from build123d import *
from build123d.topology import SkipClean

# Parameters (mm, degrees)
SKETCH3_W                 = 27
SKETCH3_H                 = 47.5
SKETCH3_R                 = 1.5
BOSS_EXTRUDE1_DEPTH       = 9
FILLET1_R                 = 2.5
SKETCH4_W                 = 26
SKETCH4_H                 = 44
BOSS_EXTRUDE5_DEPTH       = 15
SKETCH5_W                 = 25
SKETCH5_H                 = 18
BOSS_EXTRUDE6_DEPTH       = 5
SKETCH5_3_W               = 42
SKETCH5_3_H               = 18
SKETCH5_3_R               = 1
BOSS_EXTRUDE7_DEPTH       = 6
FILLET4_R                 = 2.5
CUT_EXTRUDE1_DEPTH        = 47.487229429
SKETCH6_5_R               = 22.5
BOSS_EXTRUDE8_DEPTH       = 26
SKETCH9_W                 = 7
SKETCH9_H                 = 15
SKETCH9_W_2               = 5
SKETCH9_H_2               = 6
BOSS_EXTRUDE9_DEPTH       = 7
SKETCH10_R                = 1
CUT_EXTRUDE2_DEPTH        = 41.437511922
BOSS_EXTRUDE10_DEPTH      = 5
BOSS_EXTRUDE10_DEPTH_BACK = 31
SKETCH6_6_R               = 5


with BuildPart() as part:
    # Sketch3 → Boss-Extrude1 (new body)
    with BuildSketch(Plane(origin=(0, 0, 0), x_dir=(1, 0, 0), z_dir=(0, 1, 0))):
        Rectangle(SKETCH3_W, SKETCH3_H)
        with Locations(Location((-11, 21.25, 0), (0, 0, 270))):
            Circle(SKETCH3_R, mode=Mode.SUBTRACT)
        with Locations(Location((11, 21.25, 0), (0, 0, 90))):
            Circle(SKETCH3_R, mode=Mode.SUBTRACT)
    extrude(amount=BOSS_EXTRUDE1_DEPTH)

    # Fillet1
    fillet1_edges = [part.edges().sort_by_distance(p)[0] for p in [
        (-13.5, 4.5, -23.75),
        (13.5, 4.5, -23.75),
    ]]
    fillet(fillet1_edges, radius=FILLET1_R)

    # Sketch4 → Boss-Extrude5 (add)
    with BuildSketch(Plane.XZ):
        Rectangle(SKETCH4_W, SKETCH4_H)
    extrude(amount=BOSS_EXTRUDE5_DEPTH)

    # Sketch5 → Boss-Extrude6 (add)
    with BuildSketch(Plane.XZ.offset(15)):
        with Locations((0, -0.75)):
            Rectangle(SKETCH5_W, SKETCH5_H)
    extrude(amount=-BOSS_EXTRUDE6_DEPTH)

    # Sketch5<3> → Boss-Extrude7 (add)
    with BuildSketch(Plane.XZ.offset(15)):
        with Locations((0, -0.75)):
            Rectangle(SKETCH5_3_W, SKETCH5_3_H)
        with Locations(Location((-18, -6.25, 0), (0, 0, 270))):
            Circle(SKETCH5_3_R, mode=Mode.SUBTRACT)
        with Locations(Location((18, -6.25, 0), (0, 0, 270))):
            Circle(SKETCH5_3_R, mode=Mode.SUBTRACT)
        with Locations(Location((-18, 4.75, 0), (0, 0, 270))):
            Circle(SKETCH5_3_R, mode=Mode.SUBTRACT)
        with Locations(Location((18, 4.75, 0), (0, 0, 270))):
            Circle(SKETCH5_3_R, mode=Mode.SUBTRACT)
    extrude(amount=BOSS_EXTRUDE7_DEPTH)

    # Fillet4
    fillet4_edges = [part.edges().sort_by_distance(p)[0] for p in [
        (21, -18, 8.25),
        (-21, -18, 8.25),
        (-21, -18, -9.75),
        (21, -18, -9.75),
    ]]
    fillet(fillet4_edges, radius=FILLET4_R)

    # Sketch6 → Cut-Extrude1 (cut, through all)
    with BuildSketch(Plane.ZY.offset(13)):
        with BuildLine():
            ThreePointArc((-16.66827394, -15), (-20.300466386, -7.910658998), (-21.234838924, 0))
            Line((-21.234838924, 0), (-22, 0))
            Line((-22, 0), (-22, -15))
            Line((-22, -15), (-16.66827394, -15))
        make_face()
        with BuildLine():
            Line((22, -15), (22, -9.995713029))
            ThreePointArc((22, -9.995713029), (20.719530361, -12.590758918), (19.116588355, -15))
            Line((19.116588355, -15), (22, -15))
        make_face()
    extrude(amount=-CUT_EXTRUDE1_DEPTH, mode=Mode.SUBTRACT)

    # Sketch6<5> → Boss-Extrude8 (add)
    with BuildSketch(Plane.ZY.offset(13)):
        with Locations((1.224157208, -1.357752838)):
            Circle(SKETCH6_5_R)
    extrude(amount=-BOSS_EXTRUDE8_DEPTH)

    # Sketch9 → Boss-Extrude9 (add)
    with BuildSketch(Plane.ZY.offset(13)):
        with Locations((2.25, 14)):
            Rectangle(SKETCH9_W, SKETCH9_H)
        with Locations((10.25, 9.5)):
            Rectangle(SKETCH9_W_2, SKETCH9_H_2)
    boss_extrude9 = extrude(amount=BOSS_EXTRUDE9_DEPTH)

    # Sketch10 → Cut-Extrude2 (cut, through all)
    with BuildSketch(Plane(origin=(0, 0, -1.25), x_dir=(-1, 0, 0), z_dir=(0, 0, -1))):
        with Locations((16.5, 9)):
            Circle(SKETCH10_R)
        with Locations((16.5, 19)):
            Circle(SKETCH10_R)
    cut_extrude2 = extrude(amount=-CUT_EXTRUDE2_DEPTH, mode=Mode.SUBTRACT)

    # Mirror1: Boss-Extrude9, Cut-Extrude2 across plane
    add(boss_extrude9.mirror(Plane(origin=(0, 0, 0), x_dir=(0, 0, 1), z_dir=(1, 0, 0))))
    add(cut_extrude2.mirror(Plane(origin=(0, 0, 0), x_dir=(0, 0, 1), z_dir=(1, 0, 0))), mode=Mode.SUBTRACT)

    # Sketch6<6> → Boss-Extrude10 (add, two sides: drawn at the far end of the back side and taken through both)
    with SkipClean():  # the faces are left unmerged after this step: merging them gives an invalid solid
        with BuildSketch(Plane.ZY.offset(13).offset(-BOSS_EXTRUDE10_DEPTH_BACK)):
            with Locations((1.224157208, -1.357752838)):
                Circle(SKETCH6_6_R)
        extrude(amount=BOSS_EXTRUDE10_DEPTH + BOSS_EXTRUDE10_DEPTH_BACK)


solid = part.part
Part model, mm, in its own coordinate system. A direction names the side the tool comes from. Coordinates: 2 decimals unless noted, no trailing zeros. Loops run counter-clockwise (first coordinate to the right, second up) from the corner with the lowest first, then second, coordinate; pieces in that order, holes last. Notation, with made-up numbers: (40.5, 0) -> (48.5, 0) arc R26 cw to (48.5, 29) -> close; hole circle Ø5 at (-21, -7). An arc over 180 degrees is marked (long way). Use a Markdown table: item, result. Add a question column.
Item 1: Probe probe 1 along Y at (x, z) = (16.5, 1.25); probe 2 along X at (y, z) = (-19.55, 4.75); probe 3 along Y at (x, z) = (-16.5, 2.75). List the from-to ranges inside material, lowest first.
Item 2: Band-saw the part on C-C on z = -12.5. Write the cut outline in (x, y).
Item 3: Which spindle directions (+Z, -Z, +X, -X, +Y, -Y) get a long thin tool onto all of the face, cutting with end or side? Do faces 5 (the flat face through (-16, 12.5, 10)), 6 (the cylindrical face through (-15.47, -6.24, 0.14)), 7 (the flat face through (-20, 14, 2)), 8 (the flat face through (16, -18, 8.25)). Say none if no direction does.
Item 4: Band-saw the part on D-D on y = -2. Write the cut outline in (x, z), plus the area to 3 significant figures.
Item 5: Pull direction Y, two halves, no side cores. Call faces 1 (the flat face through (16, 12.5, 10)), 2 (the flat face through (-20, 10, 10)), 3 (the flat face through (-13, -9, 1)), 4 (the flat face through (-17, -15, -1)): +Y half, -Y half, draft (parallel to the pull), parting line (faces both ways), or undercut.
Item 6: Flat gauge pins, fed straight in: P1, Ø12, axis at y = -1, z = -4.5, coming from the -X side; P2, Ø12, axis at y = 10.5, z = 2.5, coming from the +X side; P3, Ø5, axis at y = -2, z = 2, coming from the +X side; P4, Ø1.6, axis at x = -16.5, y = 9, coming from the -Z side. Where does each tip first touch, or does it go through?
Item 7: Band-saw the part on A-A on y = 19. Write the cut outline in (x, z).
Item 8: Band-saw the part on B-B on y = -19. Write the cut outline in (x, z).
Geometry says:
| question | item | result |
|---|---|---|
| 1 | probe 1 | -21 to -15, -6.36 to 3.64, 6.5 to 8, 10 to 18, 20 to 21.5 |
| 1 | probe 2 | -21 to -19, -17 to 17, 19 to 21 |
| 1 | probe 3 | -21 to -15, -6.12 to 3.4, 6.5 to 8, 10 to 18, 20 to 21.5 |
| 2 | outline | (-13.5, 0) -> (-13, 0) -> (-13, -19.19) -> (13, -19.19) -> (13, 0) -> (13.5, 0) -> (13.5, 9) -> (13, 9) -> (13, 16.47) -> (-13, 16.47) -> (-13, 9) -> (-13.5, 9) -> close |
| 3 | face 5 | +Z, -X, +Y |
| 3 | face 6 | -X |
| 3 | face 7 | +Z, -Z, -X, +Y |
| 3 | face 8 | +Z, +X, -Y |
| 4 | outline | (-18, -3.73) -> (-13, -3.73) -> (-13, -21.27) -> (13, -21.27) -> (13, -3.73) -> (18, -3.73) -> (18, 6.18) -> (13, 6.18) -> (13, 23.71) -> (-13, 23.71) -> (-13, 6.18) -> (-18, 6.18) -> close |
| 4 | area | 1,270 mm² |
| 5 | face 1 | +Y half |
| 5 | face 2 | draft |
| 5 | face 3 | undercut |
| 5 | face 4 | undercut |
| 6 | P1 | x = -18 |
| 6 | P2 | x = 20 |
| 6 | P3 | x = 18 |
| 6 | P4 | through |
| 7 | outline | (-20, -1.25) -> (-17.5, -1.25) -> (-17.5, 5.75) -> (-20, 5.75) -> close; (-15.5, -1.25) -> (-13, -1.25) -> (-13, -8.36) -> (13, -8.36) -> (13, -1.25) -> (15.5, -1.25) -> (15.5, 5.75) -> (13, 5.75) -> (13, 10.81) -> (-13, 10.81) -> (-13, 5.75) -> (-15.5, 5.75) -> close; (17.5, -1.25) -> (20, -1.25) -> (20, 5.75) -> (17.5, 5.75) -> close |
| 8 | outline | (-21, -7.25) arc R2.5 ccw to (-18.5, -9.75) -> (-13, -9.75) -> (-13, -12.74) -> (13, -12.74) -> (13, -9.75) -> (18.5, -9.75) arc R2.5 ccw to (21, -7.25) -> (21, 5.75) arc R2.5 ccw to (18.5, 8.25) -> (13, 8.25) -> (13, 15.19) -> (-13, 15.19) -> (-13, 8.25) -> (-18.5, 8.25) arc R2.5 ccw to (-21, 5.75) -> close; hole circle Ø2 at (-18, -6.25); hole circle Ø2 at (-18, 4.75); hole circle Ø2 at (18, -6.25); hole circle Ø2 at (18, 4.75) |
